Verification items for this drawing (mm, ordinates from the low corner). A direction names the side the tool comes from. Round coordinates to 2 decimals unless told otherwise and drop trailing zeros. Loops run counter-clockwise (first coordinate to the right, second up) from the corner with the lowest first, then second, coordinate; pieces in that order, holes last. Notation, with made-up numbers: M 1,11.5 L 21,11.5 A17 ccw 21,23.5 Z; hole C 26,50.5 d7. An arc over 180 degrees is marked long. One line per item, written item: value.
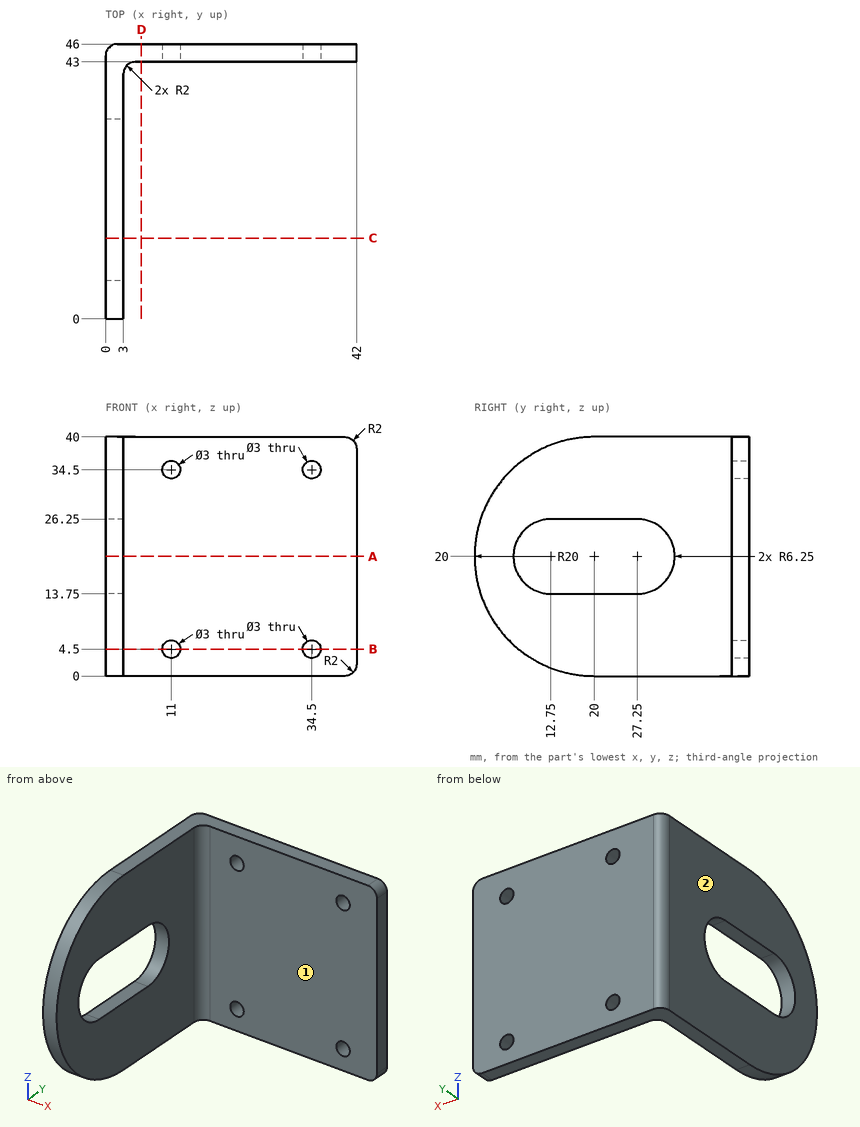
(1) Thickness scan on L1, parallel to X at y = 44, z = 4.5; L2, parallel to Y at x = 24, z = 9.5; L3, parallel to X at y = 21.5, z = 11.5. Record the ranges inside material, lowest first. Write a range as from..to.
Completed:
L1: x = 0..9.5, 12.5..33, 36..42
L2: y = 43..46
L3: x = 0..3
(2) Sectioned sample at B-B on z = 4.5. Enter the section's corners in (x, y), and give its area (3 significant figures).
Completed:
outline: M 0,7.36 L 3,7.36 L 3,41 A2 cw 5,43 L 9.5,43 L 9.5,46 L 2,46 A2 ccw 0,44 Z; M 12.5,43 L 33,43 L 33,46 L 12.5,46 Z; M 36,43 L 42,43 L 42,46 L 36,46 Z
area: 215 mm^2
(3) Sectioned sample at A-A on z = 20. Enter the section's corners in (x, y), and give its area (3 significant figures).
Completed:
outline: M 0,0 L 3,0 L 3,6.5 L 0,6.5 Z; M 0,33.5 L 3,33.5 L 3,41 A2 cw 5,43 L 42,43 L 42,46 L 2,46 A2 ccw 0,44 Z
area: 174 mm^2
(4) Tool access check on the marked faces 1 and 2. Record the directions out of +Z, -Z, +X, -X, +Y, -Y that give a thin tool (end or side, any length) a straight path to the whole face; none if there is none.
Completed:
face 1: +Z, -Z, +X, -Y
face 2: +Z, -Z, -X, +Y, -Y
(5) Depth check by flat-ended pin: pin 1 Ø2 at (y, z) = (16, 35.5) entering from +X; pin 2 Ø1.5 at (x, z) = (24.5, 5) entering from -Y; pin 3 Ø12 at (x, y) = (4.5, 11.5) entering from -Z. Enter the tip coordinate at first touch or a pass-through.
Completed:
pin 1: stops at x = 3
pin 2: stops at y = 43
pin 3: stops at z = 0.18
(6) Sectioned sample at C-C on y = 13.5. Enter the section's corners in (x, z).
Completed:
outline: M 0,1.09 L 3,1.09 L 3,13.75 L 0,13.75 Z; M 0,26.25 L 3,26.25 L 3,38.91 L 0,38.91 Z
(7) Sectioned sample at D-D on x = 6. Enter the section's corners in (y, z), and give its area (3 significant figures).
Completed:
outline: M 43,0 L 46,0 L 46,40 L 43,40 Z
area: 120 mm^2
